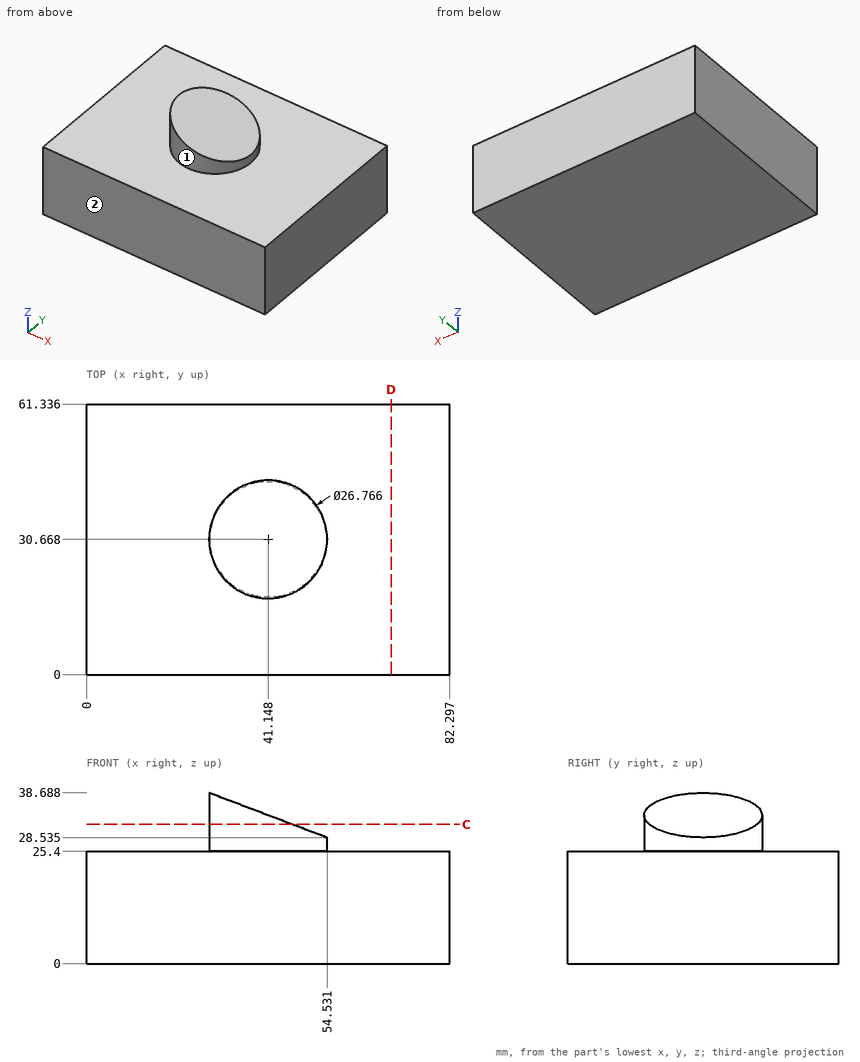
The drawing under review shows one solid part. Ordinate dimensions are in mm from its lowest x, y, z. A direction names the side the tool comes from. Round coordinates to 2 decimals unless told otherwise and drop trailing zeros. Loops run counter-clockwise (first coordinate to the right, second up) from the corner with the lowest first, then second, coordinate; pieces in that order, holes last. Notation, with made-up numbers: M -36.5,1 L -13.5,1 A24 cw -13.5,26 Z; hole C 31,57 d8. An arc over 180 degrees is marked long. Answer as CSV lines item,"result". Start each with the question number.
Item 1: Wall thickness on line 1 (Z direction, x = 42, y = 54); line 2 (X direction, y = 35, z = 28) (1 decimal); line 3 (Y direction, x = 39, z = 32.5): over which ranges is each line inside the solid? List them lowest first. Write a range as [from, to].
Item 2: Consider section D-D (x = 69). Write out the cut boundary in (y, z), then the cut area to 3 significant figures.
Item 3: Consider section C-C (z = 31.5). Write out the cut boundary in (x, y) (1 decimal).
Item 4: For the marked faces 1 and 2, list the 3-axis set-ups (+Z, -Z, +X, -X, +Y, -Y) from which the entire face can be reached by the end or side of a thin tool; tool diameter is ignored.
Item 5: Insertion check: P1, Ø12, axis at y = 14.5, z = 32.5, coming from the +X side. The pin has a flat end and moves straight along its axis. Give the tip position at first contact, or say it passes through.
Answer:
1,line 1,"z = [0, 25.4]"
1,line 2,"x = [28.5, 53.8]"
1,line 3,"y = [17.46, 43.88]"
2,outline,"M 0,0 L 61.34,0 L 61.34,25.4 L 0,25.4 Z"
2,area,"1,560 mm^2"
3,outline,"M 46.7,18.5 L 46.7,42.8 A13.4 ccw long Z"
4,face 1,"+Z"
4,face 2,"+Z, -Z, +X, -X, -Y"
5,P1,"stops at x = 49.42"
